Autodesk Inventor part; units mm, degrees
ref_plane "YZ Plane" through (0, 0, 0) normal (1, 0, 0) x (0, 1, 0)
ref_plane "XZ Plane" through (0, 0, 0) normal (0, 1, 0) x (-1, 0, 0)
ref_plane "XY Plane" through (0, 0, 0) normal (0, 0, 1) x (1, 0, 0)
sketch "Sketch1" plane through (0, 0, 0) normal (0, 0, 1) x (1, 0, 0)
  circle A0 centre (0, 0) radius 15
  dimension "d0" = 30
extrude "Extrusion1" add sketch "Sketch1" along normal blind 3
sketch "Sketch2" plane through (0, 0, 3) normal (0, 0, 1) x (1, 0, 0)
  circle A0 centre (0, 0) radius 10
  dimension "d3" = 20
extrude "Extrusion2" add sketch "Sketch2" along normal blind 18.18
sketch "Sketch3" plane through (0, 0, 21.18) normal (0, 0, 1) x (1, 0, 0)
  circle A0 centre (0, 0) radius 9
  dimension "d6" = 18
extrude "Extrusion3" add sketch "Sketch3" along normal blind 18.8
sketch "Sketch4" plane through (0, 0, 39.98) normal (0, 0, 1) x (1, 0, 0)
  circle A0 centre (0, 0) radius 8
  dimension "d9" = 16
extrude "Extrusion4" add sketch "Sketch4" along normal blind 18.8
sketch "Sketch5" plane through (0, 0, 58.78) normal (0, 0, 1) x (1, 0, 0)
  circle A0 centre (0, 0) radius 7
  dimension "d12" = 14
extrude "Extrusion5" add sketch "Sketch5" along normal blind 18.8
sketch "Sketch6" plane through (0, 0, 77.58) normal (0, 0, 1) x (1, 0, 0)
  circle A0 centre (0, 0) radius 6
  dimension "d15" = 12
extrude "Extrusion6" add sketch "Sketch6" along normal blind 18.8
sketch "Sketch7" plane through (0, 0, 96.38) normal (0, 0, 1) x (1, 0, 0)
  circle A0 centre (0, 0) radius 5
  dimension "d18" = 10
extrude "Extrusion7" add sketch "Sketch7" along normal blind 3.62
sketch "Sketch8" plane through (0, 0, 0) normal (0, 0, -1) x (-1, 0, 0)
  circle A0 centre (0, 0) radius 20
  dimension "d21" = 40
extrude "Extrusion8" cut sketch "Sketch8" against normal blind 5
sketch "Sketch9" plane through (0, 0, 5) normal (0, 0, -1) x (-1, 0, 0)
  circle A0 centre (0, 0) radius 1.75
  dimension "d24" = 3.5
extrude "Extrusion9" cut sketch "Sketch9" against normal blind 30
properties part number "Guide"
Can you work these out from the model? Positions are in its coordinate system, mm. A direction names the side the tool comes from. Round coordinates to 2 decimals unless told otherwise and drop trailing zeros. Loops run counter-clockwise (first coordinate to the right, second up) from the corner with the lowest first, then second, coordinate; pieces in that order, holes last. Notation, with made-up numbers: (29.25, 16) -> (40.25, 16) arc R16 ccw to (40.25, 23) -> close; hole circle Ø5 at (60, 82.5). An arc over 180 degrees is marked (long way). Answer in a Markdown table with one row per item.
Item 1: Suppose I cut it at B-B, the plane z = 15. List the corners of the cut face in (x, y) for me.
Answer block:
| item | result |
|---|---|
| outline | circle Ø20 at (0, 0); hole circle Ø3.5 at (0, 0) |
Item 2: On a 3-axis mill with a long thin cutter (end or side, diameter ignored), from which of +Z, -Z, +X, -X, +Y, -Y can I reach the whole of each face in a straight line? I mean faces 1 (the flat face through (0, 0, 100)), 2 (the cylindrical face through (-1.617, -0.67, 19.79)), 3 (the cylindrical face through (-6, 0, 87)). Say none if no direction works.
Answer block:
| item | result |
|---|---|
| face 1 | +Z, +X, -X, +Y, -Y |
| face 2 | -Z |
| face 3 | +Z |
Item 3: Suppose I cut it at A-A, the plane x = 0. List the corners of the cut face in (y, z) for me, plus the area to 3 significant figures.
Answer block:
| item | result |
|---|---|
| outline | (-10, 5) -> (-1.75, 5) -> (-1.75, 35) -> (1.75, 35) -> (1.75, 5) -> (10, 5) -> (10, 21.18) -> (9, 21.18) -> (9, 39.98) -> (8, 39.98) -> (8, 58.78) -> (7, 58.78) -> (7, 77.58) -> (6, 77.58) -> (6, 96.38) -> (5, 96.38) -> (5, 100) -> (-5, 100) -> (-5, 96.38) -> (-6, 96.38) -> (-6, 77.58) -> (-7, 77.58) -> (-7, 58.78) -> (-8, 58.78) -> (-8, 39.98) -> (-9, 39.98) -> (-9, 21.18) -> (-10, 21.18) -> close |
| area | 1,380 mm² |
Item 4: Suppose I cut it at D-D, the plane z = 28. List the corners of the cut face in (x, y) for me.
Answer block:
| item | result |
|---|---|
| outline | circle Ø18 at (0, 0); hole circle Ø3.5 at (0, 0) |
Item 5: Suppose I cut it at C-C, the plane z = 48. List the corners of the cut face in (x, y) for me, plus the area to 3 significant figures.
Answer block:
| item | result |
|---|---|
| outline | circle Ø16 at (0, 0) |
| area | 201 mm² |
Item 6: If I drill on probe 1 along Y at (x, z) = (0, 26.5); probe 2 along Y at (x, z) = (0, 14.5); probe 3 along X at (y, z) = (0.5, 22), over which ranges is the centre line in solid material (lowest first)?
Answer block:
| item | result |
|---|---|
| probe 1 | -9 to -1.75, 1.75 to 9 |
| probe 2 | -10 to -1.75, 1.75 to 10 |
| probe 3 | -8.99 to -1.68, 1.68 to 8.99 |
Item 7: We'd pull the mould along Y, two halves only. Please class faces 4 (the flat face through (-9, 2, 21.18)), 5 (the flat face through (0, 0, 35)), 6 (the cylindrical face through (-2.17, 9.76, 12.98)): released by +Y, released by -Y, zero draft, split by the parting line, or undercut.
Answer block:
| item | result |
|---|---|
| face 4 | zero draft |
| face 5 | undercut |
| face 6 | split by the parting line |
Item 8: Will these pins go through, and if not, where does the flat tip stop? P1, Ø1.8, axis at x = -0.5, y = 0.5, coming from the -Z side; P2, Ø10, axis at x = -2.5, z = 27.5, coming from the +Y side; P3, Ø3, axis at y = -8, z = 33, coming from the +X side.
Answer block:
| item | result |
|---|---|
| P1 | z = 35 |
| P2 | y = 9 |
| P3 | x = 6.22 |
